Work out the finished part from the listing and answer in its coordinate system (mm). A direction names the side the tool comes from. Coordinates: 2 decimals unless noted, no trailing zeros. Order: outer loops, then holes, each group sorted by start corner. A loop starts at its lowest first (then second) coordinate and runs counter-clockwise, first axis right, second up. Notation, with made-up numbers: (82, -35) - (118, -35) arc R11 cw to (118, -31) - close; hole circle Ø4 at (-0.75, 19.5). An arc over 180 degrees is marked (long way). Use CSV: the item, a comma, the result in double quotes. Start each with the question number.
from build123d import *

# Parameters (mm, degrees)
F0_W      = 57.15
F0_H      = 63.5
F1_DEPTH  = 107.95
F2_W      = 6.35
F2_H      = 6.35
F3_DEPTH  = 57.151
F4_W      = 107.95
F4_H      = 31.75
F5_DEPTH  = 31.75
F6_W      = 63.5
F6_H      = 12.7
F7_DEPTH  = 31.75
F8_W      = 63.5
F8_H      = 12.7
F9_DEPTH  = 57.151
F10_W     = 50.8
F10_H     = 6.35
F11_DEPTH = 31.75
F12_W     = 12.7
F12_H     = 50.8
F13_DEPTH = 25.401
F15_DEPTH = 63.501
F17_DEPTH = 25.401
F18_R     = 6.35
F19_DEPTH = 25.401


with BuildPart() as f1:
    # F0 (on Right) → F1 (new body)
    with BuildSketch(Plane.YZ):
        with Locations((28.575, 31.75)):
            Rectangle(F0_W, F0_H)
    extrude(amount=F1_DEPTH)

    # F2 (on face) → F3 (cut, through all)
    with BuildSketch(Plane.XZ):
        with Locations((3.175, 3.175)):
            Rectangle(F2_W, F2_H)
    extrude(amount=-F3_DEPTH, mode=Mode.SUBTRACT)

    # F4 (on face) → F5 (cut)
    with BuildSketch(Plane.XZ):
        with Locations((53.975, 47.625)):
            Rectangle(F4_W, F4_H)
    extrude(amount=-F5_DEPTH, mode=Mode.SUBTRACT)

    # F6 (on face) → F7 (cut)
    with BuildSketch(Plane.XZ):
        with Locations((76.2, 25.4)):
            Rectangle(F6_W, F6_H)
    extrude(amount=-F7_DEPTH, mode=Mode.SUBTRACT)

    # F8 (on face) → F9 (cut, through all)
    with BuildSketch(Plane.XZ):
        with Locations((76.2, 6.35)):
            Rectangle(F8_W, F8_H)
    extrude(amount=-F9_DEPTH, mode=Mode.SUBTRACT)

    # F10 (on face) → F11 (cut)
    with BuildSketch(Plane.XZ):
        with Locations((82.55, 15.875)):
            Rectangle(F10_W, F10_H)
    extrude(amount=-F11_DEPTH, mode=Mode.SUBTRACT)

    # F12 (on face) → F13 (cut, through all)
    with BuildSketch(Plane.XZ.offset(-31.75)):
        with Locations((101.6, 38.1)):
            Rectangle(F12_W, F12_H)
    extrude(amount=-F13_DEPTH, mode=Mode.SUBTRACT)

    # F14 (on face) → F15 (cut, through all)
    with BuildSketch(Plane.XY.offset(63.5)):
        Polygon((82.55, 57.15), (95.25, 41.275), (95.25, 57.15), align=None)
    extrude(amount=-F15_DEPTH, mode=Mode.SUBTRACT)

    # F16 (on face) → F17 (cut, through all)
    with BuildSketch(Plane.XZ.offset(-31.75)):
        Polygon((95.25, 63.5), (50.8, 63.5), (95.25, 31.75), align=None)
    extrude(amount=-F17_DEPTH, mode=Mode.SUBTRACT)

    # F18 (on face) → F19 (cut, through all)
    with BuildSketch(Plane.XZ.offset(-31.75)):
        with Locations((19.05, 50.8)):
            Circle(F18_R)
    extrude(amount=-F19_DEPTH, mode=Mode.SUBTRACT)


solid = f1.part
1) For faces 1 (the face through (22, 16, 31.75)), 2 (the face through (44.45, 28, 6)), 3 (the face through (57.15, 16, 16)), 4 (the face through (44.45, 16, 25)), determine the directions among +Z, -Z, +X, -X, +Y, -Y from which every point of the face is accessible in a straight line to the end or side of a thin tool.
2) Straight lines are drawn through the part: line 1 (Z direction, x = 19, y = 38); line 2 (X direction, y = 3.5, z = 17); line 3 (Y direction, x = 48.5, z = 43.5). For each, find the intervals that lie inside material, in ascending order. Write a range as [from, to].
3) The part is cut by section A-A on x = 19.05. Determine the outline of the cut face in (y, z).
4) For a pull along Z with two mould halves and no side action, classify faces 5 (the face through (6.35, 28, 3)), 6 (the face through (22.464, 44.272, 56.154)), 7 (the face through (3, 28, 6.35)), 8 (the face through (51, 16, 19.05)) as +Z half, -Z half, draft (parallel to the pull), parting line (faces both ways), or undercut.
5) Flat-ended cylindrical pins translate along their axes: P1, Ø7, axis at x = 2, y = 33.5, coming from the -Z side; P2, Ø3, axis at y = 13.5, z = 14.5, coming from the +X side; P3, Ø10, axis at x = 73.5, z = 13.5, coming from the -Y side; P4, Ø1, axis at y = 45, z = 26, coming from the -X side. Find the tip coordinate at first contact, or state that the pin passes through.
6) The part is cut by section B-B on y = 40. Determine the outline of the cut face in (x, z).
7) The part is cut by section D-D on y = 8. Determine the outline of the cut face in (x, z).
8) The part is cut by section C-C on z = 50.8. Determine the outline of the cut face in (x, y).
Answer key:
1,face 1,"+Z, +X, -X, -Y"
1,face 2,"-Z, +X, +Y, -Y"
1,face 3,"+Z, -Z, +X, -Y"
1,face 4,"+Z, +X, -Y"
2,line 1,"[0, 44.45], [57.15, 63.5]"
2,line 2,"[0, 57.15]"
2,line 3,"[31.75, 57.15]"
3,outline,"(0, 0) - (57.15, 0) - (57.15, 44.45) - (31.75, 44.45) - (31.75, 31.75) - (0, 31.75) - close; (31.75, 57.15) - (57.15, 57.15) - (57.15, 63.5) - (31.75, 63.5) - close"
4,face 5,"draft"
4,face 6,"undercut"
4,face 7,"-Z half"
4,face 8,"+Z half"
5,P1,"z = 6.35"
5,P2,"x = 57.15"
5,P3,"y = 31.75"
5,P4,"x = 0"
6,outline,"(0, 6.35) - (6.35, 6.35) - (6.35, 0) - (44.45, 0) - (44.45, 12.7) - (95.25, 12.7) - (95.25, 31.75) - (50.8, 63.5) - (0, 63.5) - close; hole circle Ø12.7 at (19.05, 50.8)"
7,outline,"(0, 6.35) - (6.35, 6.35) - (6.35, 0) - (44.45, 0) - (44.45, 12.7) - (57.15, 12.7) - (57.15, 19.05) - (44.45, 19.05) - (44.45, 31.75) - (0, 31.75) - close"
8,outline,"(0, 31.75) - (12.7, 31.75) - (12.7, 57.15) - (0, 57.15) - close; (25.4, 31.75) - (68.58, 31.75) - (68.58, 57.15) - (25.4, 57.15) - close"
